Source: CAD feature listing. Evaluate the final solid. Frame: model axes, mm. A direction names the side the tool comes from. Give positions to 0.01 mm unless a question says otherwise; leave off trailing zeros. Loops run counter-clockwise (first coordinate to the right, second up) from the corner with the lowest first, then second, coordinate; pieces in that order, holes last.
```python
from build123d import *

# Parameters (mm, degrees)
SKETCH1_W             = 20
SKETCH1_H             = 16
BOSS_EXTRUDE1_DEPTH   = 11.5
M3X0_5_TAPPED_HOLE1_D = 2.5
M6_TAPPED_HOLE1_D     = 5
CUT_EXTRUDE1_DEPTH    = 16
SKETCH10_R            = 1
CUT_EXTRUDE2_DEPTH    = 2
SKETCH11_R            = 0.75
CUT_EXTRUDE3_DEPTH    = 2.5
CHAMFER1_SIZE         = 0.5


with BuildPart() as part:
    # Sketch1 → Boss-Extrude1 (new body)
    with BuildSketch(Plane(origin=(0, 0, 0), x_dir=(1, 0, 0), z_dir=(0, 1, 0))):
        with Locations((10, 8)):
            Rectangle(SKETCH1_W, SKETCH1_H)
    extrude(amount=BOSS_EXTRUDE1_DEPTH)

    # M3x0.5 Tapped Hole1 (through all)
    with Locations(Plane(origin=(0, 11.5, 0), x_dir=(1, 0, 0), z_dir=(0, 1, 0))):
        with Locations((2.5, 8)):
            Hole(M3X0_5_TAPPED_HOLE1_D / 2)

    # M6 Tapped Hole1 (through all)
    with Locations(Plane(origin=(0, 11.5, 0), x_dir=(1, 0, 0), z_dir=(0, 1, 0))):
        with Locations((15.5, 8)):
            Hole(M6_TAPPED_HOLE1_D / 2)

    # Sketch2 → Cut-Extrude1 (cut)
    with BuildSketch(Plane.XY):
        with BuildLine():
            Line((5.5436509, 4.75), (0, 4.75))
            Line((0, 4.75), (0, 3.25))
            Line((0, 3.25), (5.5436509, 3.25))
            ThreePointArc((5.5436509, 3.25), (5.45, 4), (5.5436509, 4.75))
        make_face()
        with BuildLine():
            ThreePointArc((11.55, 4), (8.877912189, 7.026496717), (5.5436509, 4.75))
            Line((5.5436509, 4.75), (5.5436509, 3.25))
            ThreePointArc((5.5436509, 3.25), (8.877912189, 0.973503283), (11.55, 4))
        make_face()
        with BuildLine():
            Line((5.5436509, 3.25), (5.5436509, 4.75))
            ThreePointArc((5.5436509, 4.75), (5.45, 4), (5.5436509, 3.25))
        make_face()
    extrude(amount=-CUT_EXTRUDE1_DEPTH, mode=Mode.SUBTRACT)

    # Sketch10 → Cut-Extrude2 (cut)
    with BuildSketch(Plane.XY):
        with Locations((18, 2)):
            Circle(SKETCH10_R)
    extrude(amount=-CUT_EXTRUDE2_DEPTH, mode=Mode.SUBTRACT)

    # Sketch11 → Cut-Extrude3 (cut)
    with BuildSketch(Plane.XY.offset(-2)):
        with Locations((18, 2)):
            Circle(SKETCH11_R)
    extrude(amount=-CUT_EXTRUDE3_DEPTH, mode=Mode.SUBTRACT)

    # Chamfer1
    chamfer1_edges = [part.edges().sort_by_distance(p)[0] for p in [
        (20, 11.5, -8),
        (10, 11.5, -16),
        (0, 1.625, -16),
        (0, 1.625, 0),
        (0, 11.5, -8),
        (10, 0, -16),
        (20, 0, -8),
        (10, 0, 0),
        (0, 0, -8),
        (10, 11.5, 0),
        (0, 8.125, -16),
        (20, 5.75, -16),
        (20, 5.75, 0),
        (0, 8.125, 0),
    ]]
    chamfer(chamfer1_edges, length=CHAMFER1_SIZE)


solid = part.part
```
(1) Section D-D, the plane x = 2.5. Return the cut outline in (y, z), then the cut area to 4 significant figures.
A:
outline: (0, -15.5) - (0.5, -16) - (3.25, -16) - (3.25, -9.25) - (0, -9.25) - close; (0, -6.75) - (3.25, -6.75) - (3.25, 0) - (0.5, 0) - (0, -0.5) - close; (4.75, -16) - (11, -16) - (11.5, -15.5) - (11.5, -9.25) - (4.75, -9.25) - close; (4.75, -6.75) - (11.5, -6.75) - (11.5, -0.5) - (11, 0) - (4.75, 0) - close
area: 134.5 mm2
(2) Section B-B, the plane y = 9.5. Return the cut outline in (x, z).
A:
outline: (0, -15.5) - (0.5, -16) - (19.5, -16) - (20, -15.5) - (20, -0.5) - (19.5, 0) - (0.5, 0) - (0, -0.5) - close; hole circle Ø2.5 at (2.5, -8); hole circle Ø5 at (15.5, -8)
(3) Mould query, pull axis X, two halves, no side actions, for faces 4 (the cylindrical face through (19, 2, -1)), 5 (the flat face through (0, 2, -8)), 6 (the flat face through (18, 2, -4.5)), 7 (the flat face through (10, 7, 0)). Classes: pulls with the +X half, pulls with the -X half, needs draft (parallel to the pull), parting line crosses it, or undercut.
A:
face 4: undercut
face 5: pulls with the -X half
face 6: undercut
face 7: needs draft
(4) Section A-A, the plane x = 15.5. Return the cut outline in (y, z).
A:
outline: (0, -15.5) - (0.5, -16) - (11, -16) - (11.5, -15.5) - (11.5, -10.5) - (0, -10.5) - close; (0, -5.5) - (11.5, -5.5) - (11.5, -0.5) - (11, 0) - (0.5, 0) - (0, -0.5) - close
(5) Section C-C, the plane z = -4.25. Return the cut outline in (x, y).
A:
outline: (0, 0.5) - (0.5, 0) - (19.5, 0) - (20, 0.5) - (20, 11) - (19.5, 11.5) - (0.5, 11.5) - (0, 11) - (0, 4.75) - (5.54, 4.75) arc R3.05 cw (long way) to (5.54, 3.25) - (0, 3.25) - close; hole circle Ø1.5 at (18, 2)
(6) Ray query, line 1 along Y through (x, z) = (8.5, -9.5); line 2 along Y through (x, z) = (4, -3.5); line 3 along Z through (x, y) = (15.5, 7.25). Return the intervals inside material, ascending.
A:
line 1: y = 0 to 0.95, 7.05 to 11.5
line 2: y = 0 to 3.25, 4.75 to 11.5
line 3: z = -16 to -10.5, -5.5 to 0
(7) Reachability of faces 1 (the flat face through (4, 3.25, -8)), 2 (the cylindrical face through (17.405, 1.544, -3.232)), 3 (the flat face through (20, 6, -8)) from +Z, -Z, +X, -X, +Y, -Y: full face, straight path, thin tool, end or side. Return the list, or none.
A:
face 1: +Z, -Z, -X
face 2: +Z
face 3: +Z, -Z, +X, +Y, -Y
(8) First-contact query: pin 1 (1.2 mm diameter, centred on x = 18, y = 2, fed in from +Z). Flat tip, straight axial feed; report the tip coordinate or a pass-through.
A:
pin 1: stops at z = -4.5
